CAD build for the part. Positions are in the model's coordinates, mm. Face numbers are marked on the shaded views. A direction names the side the tool comes from. Give positions to 0.01 mm unless a question says otherwise; leave off trailing zeros. Write each loop counter-clockwise with the first axis right and the second up, starting at its lowest first coordinate (ties: lowest second). Pieces come first, ordered by that corner, then holes. Notation, with made-up numbers: (49.5, 76) -> (98.5, 76) arc R6 ccw to (98.5, 80) -> close; hole circle Ø10 at (47, -32). An arc over 180 degrees is marked (long way). Answer as a JSON object with one key per item and string values.
Autodesk Inventor part; units mm, degrees
ref_plane "YZ Plane" through (0, 0, 0) normal (1, 0, 0) x (0, 1, 0)
ref_plane "XZ Plane" through (0, 0, 0) normal (0, 1, 0) x (-1, 0, 0)
ref_plane "XY Plane" through (0, 0, 0) normal (0, 0, 1) x (1, 0, 0)
sketch "Sketch1" plane through (0, 0, 0) normal (0, 0, 1) x (1, 0, 0)
  line L0 (0, 0) -> (12.7, 0)
  line L1 (12.7, 0) -> (12.7, 6.35)
  line L2 (12.7, 6.35) -> (0, 6.35)
  line L3 (0, 6.35) -> (0, 0)
  line L4 (-3.175, -59.7408) -> (15.875, -59.7408)
  line L5 (15.875, -59.7408) -> (15.875, -66.0908)
  line L6 (15.875, -66.0908) -> (-3.175, -66.0908)
  line L7 (-3.175, -66.0908) -> (-3.175, -59.7408)
  line L8 (-9.525, -59.7408) -> (22.225, -59.7408) construction
  line L9 (15.875, -59.7408) -> (-3.175, -66.0908) construction
  line L10 (-3.175, -59.7408) -> (15.875, -66.0908) construction
  line L11 (6.35, -62.9158) -> (15.875, -62.9158) construction
  point P0 (6.35, 6.35)
  point P1 (6.35, -59.7408)
  dimension "d0" = 12.7
  dimension "d1" = 6.35
  dimension "d2" = 6.35
  dimension "d3" = 31.75
  dimension "d4" = 69.2658
  dimension "d5" = 6.35
  dimension "d6" = 6.35
extrude "Extrusion1" add sketch "Sketch1" along normal blind 34.29
sketch "Sketch2" plane through (0, 0, 34.29) normal (0, 0, 1) x (1, 0, 0)
  line L0 (-6.35, 6.35) -> (19.05, 6.35)
  line L1 (19.05, 6.35) -> (19.05, -78.8924)
  line L2 (19.05, -78.8924) -> (-6.35, -78.8924)
  line L3 (-6.35, -78.8924) -> (-6.35, 6.35)
  line L4 (0, 0) -> (12.7, 0)
  line L5 (12.7, 0) -> (12.7, 6.35)
  line L6 (12.7, 6.35) -> (0, 6.35)
  line L7 (0, 6.35) -> (0, 0)
  point P0 (6.35, 6.35)
  point P1 (6.35, 6.35)
  dimension "d9" = 25.4
  dimension "d10" = 85.2424
extrude "Extrusion2" add sketch "Sketch2" along normal blind 6.35
sketch "Sketch3" plane through (0, 0, 34.29) normal (0, 0, -1) x (-1, 0, 0)
  line L0 (-15.875, -66.0908) -> (-15.875, -59.7408)
  line L1 (-15.875, -59.7408) -> (3.175, -59.7408)
  line L2 (3.175, -59.7408) -> (3.175, -66.0908)
  line L3 (3.175, -66.0908) -> (-15.875, -66.0908)
  line L4 (-12.7, 0) -> (-12.7, 6.35)
  line L5 (-12.7, 6.35) -> (-19.05, 6.35)
  line L6 (-19.05, 6.35) -> (-19.05, -78.8924)
  line L7 (-19.05, -78.8924) -> (6.35, -78.8924)
  line L8 (6.35, -78.8924) -> (6.35, 6.35)
  line L9 (6.35, 6.35) -> (0, 6.35)
  line L10 (0, 6.35) -> (0, 0)
  line L11 (0, 0) -> (-12.7, 0)
  line L12 (6.35, 6.35) -> (6.35, -78.8924)
  line L13 (-19.05, -78.8924) -> (6.35, -78.8924)
  line L14 (6.35, -78.8924) -> (6.35, -72.5424)
  line L15 (6.35, -72.5424) -> (-19.05, -72.5424)
  line L16 (-19.05, -72.5424) -> (-19.05, -78.8924)
  dimension "d13" = 6.35
extrude "Extrusion3" add sketch "Sketch3" along normal blind 6.35 contours L15 L8 L7 L6
sketch "Sketch4" plane through (0, 6.35, 0) normal (0, 1, 0) x (1, 0, 0)
  line L0 (12.7, 0) -> (0, 0)
  line L1 (0, 0) -> (0, -34.29)
  line L2 (-6.35, -34.29) -> (0, -34.29)
  line L3 (-6.35, -34.29) -> (-6.35, -40.64)
  line L4 (19.05, -40.64) -> (-6.35, -40.64)
  line L5 (19.05, -34.29) -> (19.05, -40.64)
  line L6 (12.7, -34.29) -> (19.05, -34.29)
  line L7 (12.7, 0) -> (12.7, -34.29)
  line L8 (15.875, 0) -> (-3.175, 0) construction
  line L9 (6.35, 0) -> (6.35, -40.64) construction
  line L10 (-6.35, -40.64) -> (19.05, -40.64) construction
  line L11 (0, -34.29) -> (0, -40.64) construction
  line L12 (12.7, -34.29) -> (12.7, -40.64) construction
  line L13 (12.7, -40.64) -> (0, 0) construction
  line L14 (0, -40.64) -> (12.7, 0) construction
  circle A0 centre (6.35, -26.67) radius 1.5875
  circle A1 centre (6.35, -13.97) radius 1.5875
  line L15 (6.35, -20.32) -> (0, -20.32) construction
  point P0 (0, 0)
  dimension "d16" = 3.175
  dimension "d17" = 6.35
  dimension "d18" = 6.35
extrude "Extrusion4" add sketch "Sketch4" along normal blind 6.35 contours A0 | A1
sketch "Sketch5" plane through (0, 0, 40.64) normal (0, 0, 1) x (1, 0, 0)
  line L0 (19.05, 6.35) -> (-6.35, 6.35)
  line L1 (-6.35, 6.35) -> (-6.35, -78.8924)
  line L2 (-6.35, -78.8924) -> (19.05, -78.8924)
  line L3 (19.05, -78.8924) -> (19.05, 6.35)
  circle A0 centre (6.35, -33.02) radius 6.3881
  point P0 (0, 0)
  point P1 (6.35, 6.35)
  dimension "d21" = 12.7762
  dimension "d22" = 39.37
extrude "Extrusion5" cut sketch "Sketch5" against normal up to surface (6.35 mm away) contours A0
fillet "Fillet2" radius 1.27 3 edges at (6.35, 6.35, 40.64) (6.35, -78.8924, 40.64) (6.35, 6.35, 0)
equation "\"d6\" = d5"
equation "\"d18\" = d17"
properties part number "Spool Holder Cap Section Mk1"
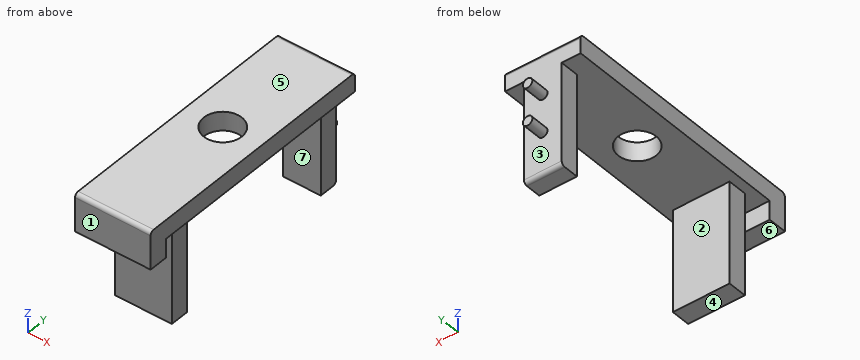
1) Pin check, flat tips, straight feed: pin 1 (5 mm diameter, centred on y = -62, z = 21.5, fed in from +X) (3 decimals); pin 2 (12 mm diameter, centred on x = 15, z = 11.5, fed in from -Y); pin 3 (5 mm diameter, centred on x = 0.5, z = 31.5, fed in from +Y). Stop position of each tip, or through.
Model answer:
{"pin 1": "stops at x = 15.875", "pin 2": "stops at y = -66.09", "pin 3": "stops at y = 6.35"}
2) Slice it at C-C (y = -33.02). List the corners of the cut face in (x, z).
Model answer:
{"outline": "(-6.35, 34.29) -> (-0.04, 34.29) -> (-0.04, 40.64) -> (-6.35, 40.64) -> close; (12.74, 34.29) -> (19.05, 34.29) -> (19.05, 40.64) -> (12.74, 40.64) -> close"}
3) Wall check: probe 1 along Y at (x, z) = (6.35, 38.25); probe 2 along X at (y, z) = (-33, 38); probe 3 along Y at (x, z) = (2.5, 19.5). Give the ranges that are in metal, low to high.
Model answer:
{"probe 1": "y = -78.89 to -39.41, -26.63 to 6.35", "probe 2": "x = -6.35 to -0.04, 12.74 to 19.05", "probe 3": "y = -66.09 to -59.74, 0 to 6.35"}
4) Mould opens along Y. For the marked faces 1, 2, 3 and 4 say: released by +Y, released by -Y, zero draft, split by the parting line, or undercut.
Model answer:
{"face 1": "released by -Y", "face 2": "undercut", "face 3": "released by +Y", "face 4": "zero draft"}
5) Slice it at B-B (x = 6.35). List the corners of the cut face in (y, z), then the cut area to 3 significant figures.
Model answer:
{"outline": "(-78.89, 27.94) -> (-72.54, 27.94) -> (-72.54, 34.29) -> (-66.09, 34.29) -> (-66.09, 0) -> (-59.74, 0) -> (-59.74, 34.29) -> (-39.41, 34.29) -> (-39.41, 40.64) -> (-77.62, 40.64) arc R1.27 ccw to (-78.89, 39.37) -> close; (-26.63, 34.29) -> (0, 34.29) -> (0, 0) -> (5.08, 0) arc R1.27 ccw to (6.35, 1.27) -> (6.35, 12.38) -> (12.7, 12.38) -> (12.7, 15.56) -> (6.35, 15.56) -> (6.35, 25.08) -> (12.7, 25.08) -> (12.7, 28.26) -> (6.35, 28.26) -> (6.35, 39.37) arc R1.27 ccw to (5.08, 40.64) -> (-26.63, 40.64) -> close", "area": "975 mm2"}
6) Slice it at D-D (z = 4). List the corners of the cut face in (x, y) (3 decimals).
Model answer:
{"outline": "(-3.175, -66.091) -> (15.875, -66.091) -> (15.875, -59.741) -> (-3.175, -59.741) -> close; (0, 0) -> (12.7, 0) -> (12.7, 6.35) -> (0, 6.35) -> close"}
7) 3-axis set-ups, long thin cutter, end or side, ignore diameter. For the marked faces 5, 6 and 7: which of +Z, -Z, +X, -X, +Y, -Y reach the whole face in a straight line?
Model answer:
{"face 5": "+Z, +X, -X, +Y, -Y", "face 6": "-Z, +X, -X, -Y", "face 7": "-Z, +X, -X"}
